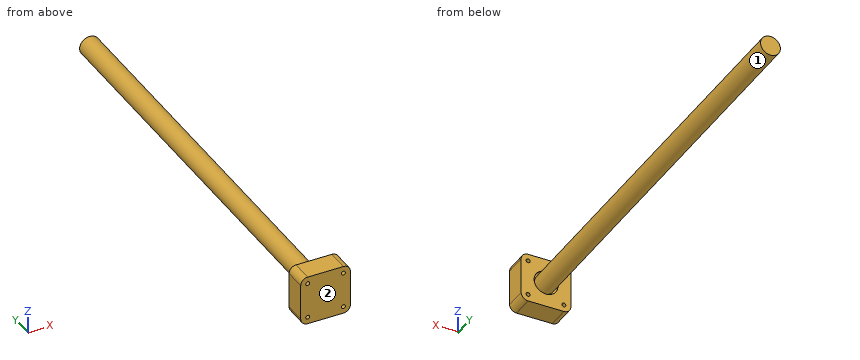
```python
from build123d import *

# Parameters (mm, degrees)
SKETCH1_W           = 50
SKETCH1_H           = 50
BOSS_EXTRUDE1_DEPTH = 22
FILLET1_R           = 7
SKETCH2_R           = 2
CUT_EXTRUDE1_DEPTH  = 22
SKETCH3_R           = 12
CUT_EXTRUDE2_DEPTH  = 3
FILLET2_R           = 2
SKETCH4_R           = 10
BOSS_EXTRUDE2_DEPTH = 430


with BuildPart() as part:
    # Sketch1 → Boss-Extrude1 (new body)
    with BuildSketch(Plane(origin=(0, 0, 0), x_dir=(1, 0, 0), z_dir=(0, 1, 0))):
        with Locations((25, -25)):
            Rectangle(SKETCH1_W, SKETCH1_H)
    extrude(amount=BOSS_EXTRUDE1_DEPTH)

    # Fillet1
    fillet1_edges = [part.edges().sort_by_distance(p)[0] for p in [
        (50, 11, 0),
        (50, 11, 50),
        (0, 11, 50),
        (0, 11, 0),
    ]]
    fillet(fillet1_edges, radius=FILLET1_R)

    # Sketch2 → Cut-Extrude1 (cut)
    with BuildSketch(Plane(origin=(0, 22, 0), x_dir=(1, 0, 0), z_dir=(0, 1, 0))):
        with Locations(Location((7, -7, 0), (0, 0, 270))):
            Circle(SKETCH2_R)
        with Locations(Location((7, -43, 0), (0, 0, 270))):
            Circle(SKETCH2_R)
        with Locations(Location((43, -43, 0), (0, 0, 270))):
            Circle(SKETCH2_R)
        with Locations(Location((43, -7, 0), (0, 0, 270))):
            Circle(SKETCH2_R)
    extrude(amount=-CUT_EXTRUDE1_DEPTH, mode=Mode.SUBTRACT)

    # Sketch3 → Cut-Extrude2 (cut)
    with BuildSketch(Plane(origin=(0, 22, 0), x_dir=(1, 0, 0), z_dir=(0, 1, 0))):
        with Locations(Location((25, -25, 0), (0, 0, 270))):
            Circle(SKETCH3_R)
    extrude(amount=-CUT_EXTRUDE2_DEPTH, mode=Mode.SUBTRACT)

    # Fillet2
    fillet2_edges = [part.edges().sort_by_distance(p)[0] for p in [
        (25, 19, 13),
    ]]
    fillet(fillet2_edges, radius=FILLET2_R)

    # Sketch4 → Boss-Extrude2 (add)
    with BuildSketch(Plane(origin=(0, 19, 0), x_dir=(1, 0, 0), z_dir=(0, 1, 0))):
        with Locations(Location((25, -25, 0), (0, 0, 270))):
            Circle(SKETCH4_R)
    extrude(amount=BOSS_EXTRUDE2_DEPTH)


solid = part.part
```
Input: part model. Units: mm. Frame: model coordinates. Face numbers are marked on the shaded views. Round coordinates to 2 decimals unless told otherwise and drop trailing zeros. Loops run counter-clockwise (first coordinate to the right, second up) from the corner with the lowest first, then second, coordinate; pieces in that order, holes last. Notation, with made-up numbers: M 6,57.5 L 25,57.5 A31 cw 25,93.5 Z; hole C -38.75,88 d6. An arc over 180 degrees is marked long. Answer in a Markdown table with one row per item. Add a question column.
1. Section B-B (x = 25). Output: boundary loops of the cut face in (y, z), and give its area (3 significant figures).
2. Contact query for flat-ended pins moving along their axis: pin 1 (5 mm diameter, centred on y = 302, z = 34.5, fed in from +X); pin 2 (3.5 mm diameter, centred on x = 43, z = 43, fed in from +Y); pin 3 (8 mm diameter, centred on x = 38.5, z = 26.5, fed in from +Y); pin 4 (5 mm diameter, centred on x = 7, z = 43, fed in from +Y). Output: stop coordinate, or through.
3. Mould query, pull axis Y, two halves, no side actions, for the marked faces 1 and 2. Classes: released by +Y, released by -Y, zero draft, split by the parting line, or undercut.
4. Section C-C (y = 272.5). Output: boundary loops of the cut face in (x, z).
5. Ray query, probe 1 along X at (y, z) = (21.45, 25); probe 2 along X at (y, z) = (7, 7); probe 3 along Y at (x, z) = (10.5, 25). Return the intervals inside material, ascending.
6. Section A-A (z = 25). Output: boundary loops of the cut face in (x, y).
Values follow:
| question | item | result |
|---|---|---|
| 1 | outline | M 0,0 L 22,0 L 22,13 L 21,13 A2 cw 19,15 L 449,15 L 449,35 L 19,35 A2 cw 21,37 L 22,37 L 22,50 L 0,50 Z |
| 1 | area | 9,630 mm^2 |
| 2 | pin 1 | x = 32.14 |
| 2 | pin 2 | through |
| 2 | pin 3 | y = 449 |
| 2 | pin 4 | y = 22 |
| 3 | face 1 | zero draft |
| 3 | face 2 | released by -Y |
| 4 | outline | C 25,25 d20 |
| 5 | probe 1 | 0 to 13, 15 to 35, 37 to 50 |
| 5 | probe 2 | 0 to 5, 9 to 41, 45 to 50 |
| 5 | probe 3 | 0 to 22 |
| 6 | outline | M 0,0 L 50,0 L 50,22 L 37,22 L 37,21 A2 cw 35,19 L 35,449 L 15,449 L 15,19 A2 cw 13,21 L 13,22 L 0,22 Z |
